Study the drawing (mm; zero at the part's minimum x, y, z) and answer. A direction names the side the tool comes from. Coordinates: 2 decimals unless noted, no trailing zeros. Order: outer loops, then holes, each group sorted by start corner. A loop starts at its lowest first (then second) coordinate and runs counter-clockwise, first axis right, second up.
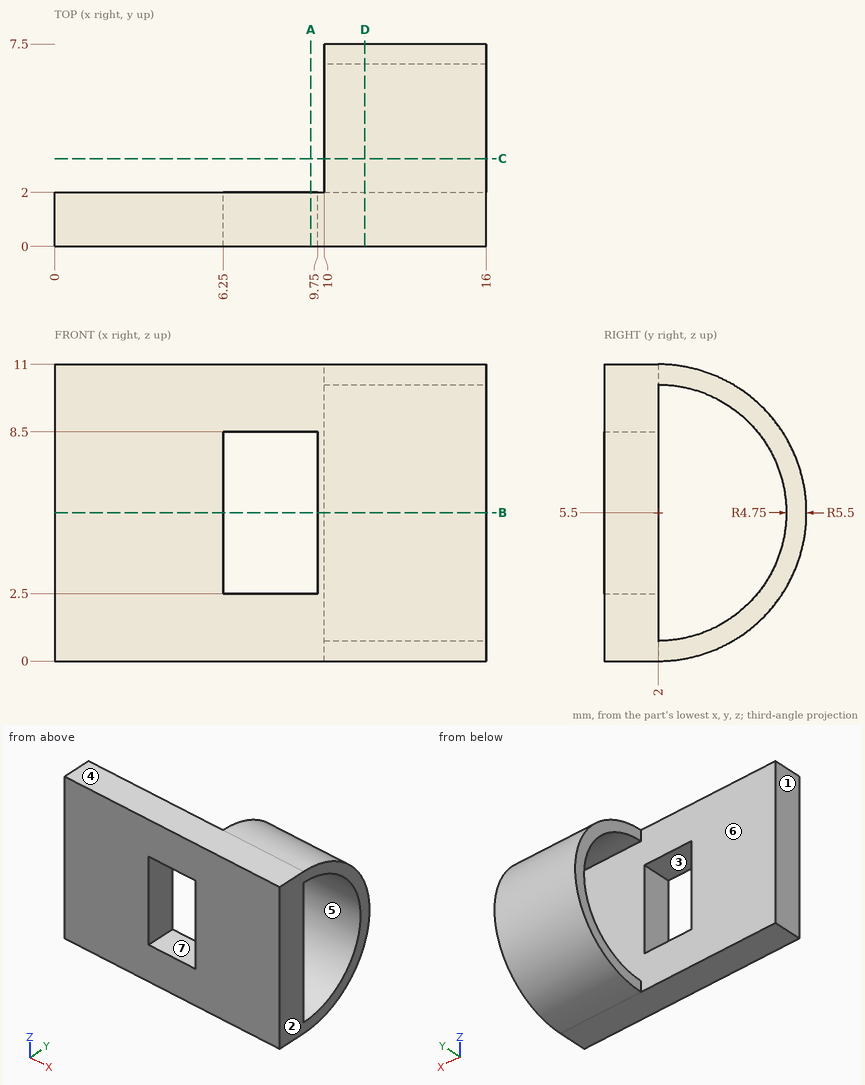
1) A cutting plane is placed at B-B, the plane z = 5.5. Determine the outline of the cut face in (x, y).
A:
outline: (0, 0) - (6.25, 0) - (6.25, 2) - (0, 2) - close; (9.75, 0) - (16, 0) - (16, 2) - (9.75, 2) - close; (10, 6.75) - (16, 6.75) - (16, 7.5) - (10, 7.5) - close
2) A cutting plane is placed at D-D, the plane x = 11.5. Determine the outline of the cut face in (y, z), and give its area (3 significant figures).
A:
outline: (0, 0) - (2, 0) arc R5.5 ccw to (2, 11) - (0, 11) - close; hole (2, 0.75) arc R4.75 ccw to (2, 10.25) - close
area: 34.1 mm2
3) Which of the six approach directions +Z, -Z, +X, -X, +Y, -Y give full straight-line access (tool end or side, diameter ignored) to the marked faces 5, 6 and 7?
A:
face 5: +X, -X
face 6: -X
face 7: +Y, -Y
4) A cutting plane is placed at C-C, the plane y = 3.25. Determine the outline of the cut face in (x, z), and give its area (3 significant figures).
A:
outline: (10, 0.14) - (16, 0.14) - (16, 0.92) - (10, 0.92) - close; (10, 10.08) - (16, 10.08) - (16, 10.86) - (10, 10.86) - close
area: 9.28 mm2
5) Determine the mould class of the marked faces 1, 2, 3 and 4 for opening direction X: pulls with the +X half, pulls with the -X half, needs draft (parallel to the pull), parting line crosses it, or undercut.
A:
face 1: pulls with the -X half
face 2: pulls with the +X half
face 3: undercut
face 4: needs draft
6) Straight lines are drawn through the part: line 1 (X direction, y = 1.75, z = 3.5); line 2 (Z direction, x = 7, y = 0.75); line 3 (Y direction, x = 5.25, z = 8.5). For each, find the intervals that lie inside material, in ascending order.
A:
line 1: x = 0 to 6.25, 9.75 to 16
line 2: z = 0 to 2.5, 8.5 to 11
line 3: y = 0 to 2
7) A flat-ended cylindrical pin translates along its axis: pin 1 Ø5 at (x, z) = (9.5, 9.5) entering from +Y. Find the tip coordinate at first contact, or state that the pin passes through.
A:
pin 1: stops at y = 7.28
8) A cutting plane is placed at A-A, the plane x = 9.5. Determine the outline of the cut face in (y, z), and give its area (3 significant figures).
A:
outline: (0, 0) - (2, 0) - (2, 2.5) - (0, 2.5) - close; (0, 8.5) - (2, 8.5) - (2, 11) - (0, 11) - close
area: 10.0 mm2
